Autodesk Inventor part; units mm, degrees
ref_plane "YZ Plane" through (0, 0, 0) normal (1, 0, 0) x (0, 1, 0)
ref_plane "XZ Plane" through (0, 0, 0) normal (0, 1, 0) x (-1, 0, 0)
ref_plane "XY Plane" through (0, 0, 0) normal (0, 0, 1) x (1, 0, 0)
sketch "Sketch1" plane through (0, 0, 0) normal (0, 0, 1) x (1, 0, 0)
  line L0 (0, 0) -> (0, -14.67)
  line L1 (0, -14.67) -> (-10.8, -14.67)
  line L2 (-10.8, -14.67) -> (-12, -8.67)
  line L3 (-12, -8.67) -> (-12, 9.98)
  line L4 (-12, 9.98) -> (-8.4, 9.98)
  line L5 (-8.4, 9.98) -> (-8.4, 0)
  line L6 (-8.4, 0) -> (0, 0)
  dimension "d0" = 24.65
  dimension "d1" = 6
  dimension "d2" = 12
  dimension "d3" = 8.4
  dimension "d4" = 14.67
  dimension "d5" = 10.8
extrude "Extrusion1" add sketch "Sketch1" along normal blind 6.75
sketch "Sketch2" plane through (0, 0, 6.75) normal (0, 0, 1) x (1, 0, 0)
  line L0 (0, -14.67) -> (0, 0)
  line L1 (0, 0) -> (-8.4, 0)
  line L2 (-8.4, 0) -> (-8.4, 9.98)
  line L3 (-8.4, 9.98) -> (-12, 9.98)
  line L4 (-12, 9.98) -> (-12, -8.67)
  line L5 (-12, -8.67) -> (-10.8, -14.67)
  line L6 (-10.8, -14.67) -> (0, -14.67)
  line L7 (-12, 9.98) -> (-8.4, 9.98)
  line L8 (-8.4, 9.98) -> (-8.4, 4.58)
  line L9 (-8.4, 4.58) -> (-12, 4.58)
  line L10 (-12, 4.58) -> (-12, 9.98)
  dimension "d8" = 5.4
extrude "Extrusion2" cut sketch "Sketch2" against normal blind 4.42 contours L9 L4 L3 L2
fillet "Fillet1" radius 2 1 edges at (-12, 9.98, 1.165)
sketch "Sketch3" plane through (0, 0, 6.75) normal (0, 0, 1) x (1, 0, 0)
  line L0 (-12, 4.58) -> (-12, -8.67)
  line L1 (-10.8, -14.67) -> (0, -14.67)
  line L2 (-8.4, 4.58) -> (-12, 4.58)
  point P0 (0, 0)
  point P1 (-9.59, -12.45)
  point P2 (-10.1, -1.02)
  point P3 (-10.1, 6.36)
  dimension "d13" = 1.9
  dimension "d14" = 1.9
  dimension "d15" = 2.22
  dimension "d26" = 5.6
  dimension "d27" = 1.78
  dimension "d28" = 1.21
hole "Hole1" at (-9.59, -12.45, 6.75) at (-10.1, -1.02, 6.75) at (-10.1, 6.36, 6.75) direction (0, 0, -1) diameter 1.45 end through all
sketch "Sketch4" plane through (0, 0, 6.75) normal (0, 0, 1) x (1, 0, 0)
  line L0 (0, -14.67) -> (0, 0)
  line L1 (0, -6.52) -> (-1.87, -4.65)
  line L2 (-1.87, -4.65) -> (-1.87, 0)
  line L3 (0, 0) -> (-8.4, 0)
  line L4 (0, -13.46) -> (-1.21, -14.67)
  line L5 (-10.8, -14.67) -> (0, -14.67)
  dimension "d29" = 1.87
  dimension "d30" = 135
  dimension "d31" = 1.21
  dimension "d32" = 1.21
  dimension "d34" = 4.65
extrude "Extrusion3" cut sketch "Sketch4" against normal blind 1.8
sketch "Sketch5" plane through (0, 0, 6.75) normal (0, 0, 1) x (1, 0, 0)
  line L0 (-10.8, -14.67) -> (-1.21, -14.67)
  line L1 (-1.21, -14.67) -> (-1.21, -16.67)
  line L2 (-1.21, -16.67) -> (-3.21, -18.67)
  line L3 (-3.21, -18.67) -> (-10, -18.67)
  line L4 (-12, -8.67) -> (-10.8, -14.67)
  line L5 (-10, -18.67) -> (-10.8, -14.67)
  point P0 (0, 0)
  dimension "d37" = 4
  dimension "d38" = 135
  dimension "d39" = 2
extrude "Extrusion4" add sketch "Sketch5" against normal blind 0.7
ref_plane "Work Plane1" through (-2.91, -16.67, 6.75) normal (1, 0, 0) x (0, 0, -1)
sketch "Sketch6" plane through (-2.91, -16.67, 6.75) normal (1, 0, 0) x (0, 0, -1)
  line L0 (0.7, 2) -> (0.7, -0.6)
  line L1 (0.7, 2) -> (0.7, 0)
  line L2 (0.7, 2) -> (4.5, 2)
  line L3 (4.5, 2) -> (0.7, -0.6)
  line L4 (0.7, 2) -> (0.7, 0)
  line L5 (6.75, 2) -> (1.8, 2)
  point P0 (6.75, 16.87)
  dimension "d42" = 3.8
  dimension "d43" = 2.6
extrude "Extrusion5" add sketch "Sketch6" against normal blind 0.7
pattern_linear "Rectangular Pattern1" count 3 spacing 3 along (-1, 0, 0) of "Extrusion5"
sketch "Sketch7" plane through (0, 0, 6.75) normal (0, 0, 1) x (1, 0, 0)
  circle A0 centre (-2.8, -15.87) radius 0.5
  circle A1 centre (-10.25, 2.28) radius 0.5
  line L0 (-12, 4.58) -> (-12, -8.67)
  line L1 (-8.4, 4.58) -> (-12, 4.58)
  line L2 (-1.21, -14.67) -> (-1.21, -16.67)
  line L3 (0, -14.67) -> (-1.21, -14.67)
  line L4 (-3.21, -18.67) -> (-10, -18.67)
  line L5 (0, -13.46) -> (0, -6.52)
  point P0 (0, 0)
  dimension "d50" = 1
  dimension "d51" = 1
  dimension "d85" = 1.25
  dimension "d86" = 1.8
  dimension "d87" = 2.3
  dimension "d88" = 2.3
extrude "Extrusion6" add sketch "Sketch7" along normal blind 1.05
fillet "Fillet2" radius 0.2 2 edges at (-3.3, -15.87, 7.8) (-10.75, 2.28, 7.8)
sketch "Sketch8" plane through (0, 0, 6.75) normal (0, 0, 1) x (1, 0, 0)
  circle A0 centre (-4.4, -10.37) radius 3.9
  line L0 (0, -13.46) -> (0, -6.52)
  line L1 (-3.21, -18.67) -> (-10, -18.67)
  point P0 (0, 0)
  dimension "d59" = 7.8
  dimension "d60" = 0.5
  dimension "d61" = 4.4
extrude "Extrusion7" cut sketch "Sketch8" against normal blind 2
chamfer "Chamfer1" distance 0.2 angle 45 5 edges at (-9.59, -11.725, 0) (-10.1, -0.295, 0) (-10.1, 7.085, 0) (-9.59, -11.725, 6.75) (-10.1, -0.295, 6.75)
sketch "Sketch9" plane through (0, 0, 0) normal (0, 0, -1) x (-1, 0, 0)
  circle A0 centre (3.75, -2.92) radius 0.75
  circle A1 centre (8.39, -8.92) radius 0.75
  line L0 (0, 0) -> (0, -14.67)
  line L1 (0, -14.67) -> (10.8, -14.67)
  line L2 (12, -8.67) -> (12, 7.98)
  dimension "d67" = 1.5
  dimension "d68" = 1.5
  dimension "d69" = 3
  dimension "d70" = 11
  dimension "d71" = 5
  dimension "d72" = 2.86
extrude "Extrusion8" add sketch "Sketch9" along normal blind 1
chamfer "Chamfer2" distance 0.2 angle 45 2 edges at (-7.64, -8.92, -1) (-3, -2.92, -1)
sketch "Sketch10" plane through (-8.4, 9.98, 2.33) normal (0, 1, 0) x (1, 0, 0)
  line L0 (-1.6, 0) -> (-1.6, 2.33)
  line L1 (-1.6, 0) -> (0, 0)
  line L2 (0, 2.33) -> (0, 0)
  line L3 (-1.6, 2.33) -> (0, 2.33)
  line L4 (-1.6, 0) -> (-0.6, 0)
  line L5 (-0.6, 0) -> (-0.6, 1)
  line L6 (-0.6, 1) -> (-1.6, 1)
  line L7 (-1.6, 1) -> (-1.6, 0)
  point P0 (8.4, 2.33)
  dimension "d78" = 1
  dimension "d79" = 1
extrude "Extrusion9" add sketch "Sketch10" along normal blind 1.2 contours L0 L6 L5 L1
sketch "Sketch11" plane through (0, 0, 6.75) normal (0, 0, 1) x (1, 0, 0)
  arc A0 (-7.1046, -7.5602) -> (-8.0174, -8.9124) centre (-8.4, -7.67) ccw
  circle A1 centre (-4.4, -10.37) radius 3.9
  line L0 (-3.21, -18.67) -> (-10, -18.67)
  line L1 (-12, 4.58) -> (-12, -8.67)
  point P0 (0, 0)
  dimension "d82" = 9.7
  dimension "d83" = 2.3
  dimension "d84" = 2.6
extrude "Extrusion10" add sketch "Sketch11" along normal blind 0.25 contours A1 A0
equation "\"d32\" = d31"
equation "\"d68\" = d67"
properties part number "J024 mount"
The model under review builds one solid part; all positions refer to its coordinate system, in mm. A direction names the side the tool comes from. Give positions to 0.01 mm unless a question says otherwise; leave off trailing zeros. Write each loop counter-clockwise with the first axis right and the second up, starting at its lowest first coordinate (ties: lowest second). Pieces come first, ordered by that corner, then holes.
(1) The part is to be moulded in two halves that separate along X. For faces 6 (the flat face through (-4, 0, 3)), 7 (the flat face through (-12, -2, 3)), 8 (the flat face through (-5, -17, 6.05)), 9 (the cylindrical face through (-7.27, -7.73, 5.89)), say which applies: released by +X, released by -X, zero draft, split by the parting line, or undercut.
(2) Consider section D-D, the plane y = 2.28. Give the boundary of the cut face in (x, z).
(3) Consider section B-B, the plane z = 3.75. Give the boundary of the cut face in (x, y) (3 decimals), and give its area (3 significant figures).
(4) Consider section A-A, the plane y = -10.37. Give the boundary of the cut face in (x, z), and give its area (3 significant figures).
(5) To check wall thickness, follow L1, parallel to Y at x = -10.1, z = 2.5 (3 decimals); L2, parallel to Y at x = -10, z = 1; L3, parallel to Z at x = -4, y = -11.75. State the ranges of each line that lie inside material, in increasing order.
(6) Tool access review of faces 1 (the flat face through (-1, -2, 4.95)), 2 (the cylindrical face through (-3.2, -3.43, -0.39)), 3 (the flat face through (-10, 4.58, 5)), 4 (the flat face through (-5, -14.67, 2)), 5 (the cylindrical face through (-10.619, 1.942, 7.169)): name each direction out of +Z, -Z, +X, -X, +Y, -Y from which nothing blocks a thin tool from reaching the whole face with its end or side.
(7) For P1, Ø3.5, axis at x = -4, y = -4.5, coming from the +Z side; P2, Ø1.5, axis at x = -1, z = 2, coming from the -Y side; P3, Ø2, axis at x = -3.5, z = 6, coming from the +Y side; P4, Ø5, axis at x = -5, z = 4, coming from the -Y side, all flat-tipped, find the tip position at first contact; note any pin that passes through.
(8) Consider section C-C, the plane z = 0.75. Give the boundary of the cut face in (x, y) (3 decimals), and give its area (3 significant figures).
Returned:
1. face 6: zero draft
1. face 7: released by -X
1. face 8: undercut
1. face 9: undercut
2. outline: (-12, 0) - (-8.4, 0) - (-8.4, 6.75) - (-9.75, 6.75) - (-9.75, 7.6) arc R0.2 ccw to (-9.95, 7.8) - (-10.55, 7.8) arc R0.2 ccw to (-10.75, 7.6) - (-10.75, 6.75) - (-12, 6.75) - close
3. outline: (-12, -8.67) - (-10.8, -14.67) - (-9.61, -14.67) - (-9.61, -15.696) - (-8.91, -15.696) - (-8.91, -14.67) - (-6.61, -14.67) - (-6.61, -15.696) - (-5.91, -15.696) - (-5.91, -14.67) - (-3.61, -14.67) - (-3.61, -15.696) - (-2.91, -15.696) - (-2.91, -14.67) - (0, -14.67) - (0, 0) - (-8.4, 0) - (-8.4, 4.58) - (-12, 4.58) - close; hole circle Ø1.45 at (-10.1, -1.02); hole circle Ø1.45 at (-9.59, -12.45)
3. area: 188 mm2
4. outline: (-11.66, 0) - (0, 0) - (0, 6.75) - (-0.5, 6.75) - (-0.5, 4.75) - (-8.3, 4.75) - (-8.3, 6.75) - (-11.66, 6.75) - close
4. area: 63.1 mm2
5. L1: y = -14.67 to -12.965, -11.935 to -1.745, -0.295 to 4.58
5. L2: y = -14.67 to -13.05, -11.85 to -1.74, -0.3 to 5.64, 7.08 to 9.98
5. L3: z = 0 to 4.75
6. face 1: +Z, +X, +Y
6. face 2: -Z
6. face 3: +Z, +X, -X, +Y
6. face 4: -Z, -Y
6. face 5: +Z
7. P1: stops at z = 6.75
7. P2: stops at y = -14.67
7. P3: stops at y = 0
7. P4: stops at y = -18.67
8. outline: (-12, -8.67) - (-10.8, -14.67) - (0, -14.67) - (0, 0) - (-8.4, 0) - (-8.4, 9.98) - (-10, 9.98) arc R2 ccw to (-12, 7.98) - close; hole circle Ø1.45 at (-10.1, -1.02); hole circle Ø1.45 at (-10.1, 6.36); hole circle Ø1.45 at (-9.59, -12.45)
8. area: 203 mm2
